from build123d import *

# Parameters (mm, degrees)
F0_W     = 71.5
F0_H     = 66
F3_DEPTH = 33
F4_R     = 50
F5_DEPTH = 40.5
F6_R     = 39.5
F7_DEPTH = 28.5
F8_W     = 12.8
F8_H     = 14.5
F9_DEPTH = 60


with BuildPart() as f1:
    # F0 (on Front) → F1 (revolve)
    with BuildSketch(Plane.XZ):
        with Locations((35.75, 33)):
            Rectangle(F0_W, F0_H)
    revolve(axis=Axis((0, 0, 33), (0, 0, 1)))

    # F2 (on face) → F3 (join)
    with BuildSketch(Plane.XY.offset(66)):
        Polygon((38, 30), (30, 38), (-30, 38), (-38, 30), (-38, -30), (-30, -38), (30, -38), (38, -30), align=None)
    extrude(amount=F3_DEPTH)

    # F4 (on face) → F5 (join)
    with BuildSketch(Plane.XY.offset(99)):
        Circle(F4_R)
        Polygon((30, 38), (38, 30), (38, -30), (30, -38), (-30, -38), (-38, -30), (-38, 30), (-30, 38), align=None, mode=Mode.SUBTRACT)
        Polygon((38, -30), (38, 30), (30, 38), (-30, 38), (-38, 30), (-38, -30), (-30, -38), (30, -38), align=None)
    extrude(amount=F5_DEPTH)

    # F6 (on face) → F7 (join)
    with BuildSketch(Plane.XY.offset(139.5)):
        Circle(F6_R)
    extrude(amount=F7_DEPTH)

    # F8 (on Right) → F9 (join, symmetric)
    with BuildSketch(Plane.YZ):
        with Locations((0, 129.75)):
            Rectangle(F8_W, F8_H)
    extrude(amount=F9_DEPTH, both=True)


solid = f1.part
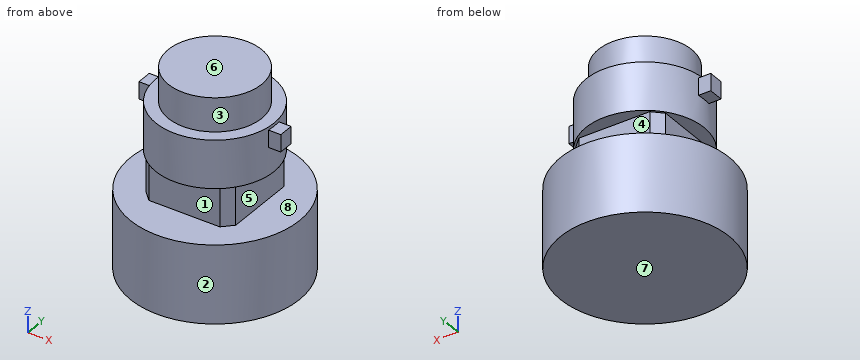
CAD build for the part. Positions are in the model's coordinates, mm. Face numbers are marked on the shaded views. A direction names the side the tool comes from. Round coordinates to 2 decimals unless told otherwise and drop trailing zeros. Write each loop counter-clockwise with the first axis right and the second up, starting at its lowest first coordinate (ties: lowest second). Pieces come first, ordered by that corner, then holes.
(1) Slice it at D-D, the plane z = 83. Write the cut outline in (x, y), and give its area (3 significant figures).
(2) Probe line 1 along Z through (x, y) = (8, -41); line 2 along Z through (x, y) = (34.5, -54); line 3 along Y through (x, z) = (-11, 91). List the from-to ranges inside material, lowest first.
(3) 3-axis set-ups, long thin cutter, end or side, ignore diameter. For the marked faces 1, 2, 3, 4 and 5: which of +Z, -Z, +X, -X, +Y, -Y reach the whole face in a straight line?
(4) Slice it at C-C, the plane y = 0. Write the cut outline in (x, z), and give its area (3 significant figures).
(5) Mould opens along Z. For the marked faces 6, 7 and 8 say: pulls with the +Z half, pulls with the -Z half, needs draft (parallel to the pull), parting line crosses it, or undercut.
(6) Slice it at A-A, the plane y = 42.5. Write the cut outline in (x, z), and give its area (3 significant figures).
(7) Drop flat-ended pins along their axis: P1, Ø3, axis at x = 45.5, z = 22, coming from the -Y side; P2, Ø5, axis at x = -46.5, y = -40, coming from the +Z side; P3, Ø16.5, axis at x = 14.5, z = 84, coming from the -Y side. Give the stop position or say it passes through.
(8) Slice it at B-B, the plane x = 0. Write the cut outline in (y, z), and give its area (3 significant figures).
From the geometry:
1. outline: (-38, -30) - (-30, -38) - (30, -38) - (38, -30) - (38, 30) - (30, 38) - (-30, 38) - (-38, 30) - close
1. area: 5,650 mm2
2. line 1: z = 0 to 66, 99 to 139.5
2. line 2: z = 0 to 66
2. line 3: y = -38 to 38
3. face 1: +X, -X, -Y
3. face 2: +Z, -Z
3. face 3: +Z
3. face 4: +X, -X, +Y
3. face 5: +X, +Y, -Y
4. outline: (-71.5, 0) - (71.5, 0) - (71.5, 66) - (38, 66) - (38, 99) - (50, 99) - (50, 122.5) - (60, 122.5) - (60, 137) - (50, 137) - (50, 139.5) - (39.5, 139.5) - (39.5, 168) - (-39.5, 168) - (-39.5, 139.5) - (-50, 139.5) - (-50, 137) - (-60, 137) - (-60, 122.5) - (-50, 122.5) - (-50, 99) - (-38, 99) - (-38, 66) - (-71.5, 66) - close
4. area: 18,500 mm2
5. face 6: pulls with the +Z half
5. face 7: pulls with the -Z half
5. face 8: undercut
6. outline: (-57.5, 0) - (57.5, 0) - (57.5, 66) - (-57.5, 66) - close; (-26.34, 99) - (26.34, 99) - (26.34, 139.5) - (-26.34, 139.5) - close
6. area: 9,720 mm2
7. P1: stops at y = -56.36
7. P2: stops at z = 66
7. P3: stops at y = -38
8. outline: (-71.5, 0) - (71.5, 0) - (71.5, 66) - (38, 66) - (38, 99) - (50, 99) - (50, 139.5) - (39.5, 139.5) - (39.5, 168) - (-39.5, 168) - (-39.5, 139.5) - (-50, 139.5) - (-50, 99) - (-38, 99) - (-38, 66) - (-71.5, 66) - close
8. area: 18,200 mm2
